from build123d import *

# Parameters (mm, degrees)
F0_R     = 1.35
F1_DEPTH = 29.5
F2_DEPTH = 37
F3_R     = 3
F4_R     = 10
F5_SIZE  = 10
F6_R     = 1.5
F7_DEPTH = 25


with BuildPart() as f1:
    # F0 (on Top) → F1 (new body)
    with BuildSketch(Plane.XY):
        with BuildLine():
            Line((-1.6, 2.8), (1.6, 2.8))
            Line((1.6, 2.8), (3.0028275917, 7.4646537393))
            ThreePointArc((3.0028275917, 7.4646537393), (0, 5.85035927), (-3.0028275917, 7.4646537393))
            Line((-3.0028275917, 7.4646537393), (-1.6, 2.8))
        make_face()
        with BuildLine():
            ThreePointArc((-3.0028275917, 7.4646537393), (0, 5.85035927), (3.0028275917, 7.4646537393))
            Line((3.0028275917, 7.4646537393), (3.6, 9.45035927))
            ThreePointArc((3.6, 9.45035927), (0, 13.05035927), (-3.6, 9.45035927))
            Line((-3.6, 9.45035927), (-3.0028275917, 7.4646537393))
        make_face()
        with Locations((0, 9.45035927)):
            Circle(F0_R, mode=Mode.SUBTRACT)
        Polygon((-15, 0), (15, 0), (15, 2.8), (1.6, 2.8), (-1.6, 2.8), (-15, 2.8), align=None)
        with BuildLine():
            ThreePointArc((-3.6, 9.45035927), (-3.4474758397, 8.4135804435), (-3.0028275917, 7.4646537393))
            Line((-3.0028275917, 7.4646537393), (-3.6, 9.45035927))
        make_face()
        with BuildLine():
            Line((3.6, 9.45035927), (3.0028275917, 7.4646537393))
            ThreePointArc((3.0028275917, 7.4646537393), (3.4474758397, 8.4135804435), (3.6, 9.45035927))
        make_face()
    extrude(amount=F1_DEPTH)

    # F0 (on Top) → F2 (join)
    with BuildSketch(Plane.XY):
        Polygon((-15, 0), (15, 0), (15, 2.8), (1.6, 2.8), (-1.6, 2.8), (-15, 2.8), align=None)
    extrude(amount=F2_DEPTH)

    # F3
    f3_edges = [f1.edges().sort_by_distance(p)[0] for p in [
        (-1.6, 2.8, 14.75),
        (1.6, 2.8, 14.75),
        (0, 2.8, 29.5),
    ]]
    fillet(f3_edges, radius=F3_R)

    # F4
    f4_edges = [f1.edges().sort_by_distance(p)[0] for p in [
        (-15, 1.4, 37),
        (15, 1.4, 37),
    ]]
    fillet(f4_edges, radius=F4_R)

    # F5
    f5_edges = [f1.edges().sort_by_distance(p)[0] for p in [
        (15, 1.4, 0),
        (-15, 1.4, 0),
    ]]
    chamfer(f5_edges, length=F5_SIZE)

    # F6 (on face) → F7 (cut)
    with BuildSketch(Plane(origin=(0, 2.8, 0), x_dir=(-1, 0, 0), z_dir=(0, 1, 0))):
        with Locations((-9, 31)):
            Circle(F6_R)
        with Locations((9, 31)):
            Circle(F6_R)
        with Locations((-9, 11)):
            Circle(F6_R)
        with Locations((9, 11)):
            Circle(F6_R)
    extrude(amount=-F7_DEPTH, mode=Mode.SUBTRACT)


solid = f1.part
Verification items for the finished model (mm, model axes). A direction names the side the tool comes from. Coordinates: 2 decimals unless noted, no trailing zeros. Write each loop counter-clockwise with the first axis right and the second up, starting at its lowest first coordinate (ties: lowest second). Pieces come first, ordered by that corner, then holes. Notation, with made-up numbers: M 33.25,88.5 L 86.25,88.5 A20 ccw 86.25,96.5 Z; hole C 27,79 d8. An arc over 180 degrees is marked long. Use a Markdown table: item, result.
Q1. Thickness scan on line 1 (Y direction, x = 0, z = 15); line 2 (Z direction, x = -9, y = 1.15); line 3 (Y direction, x = 9, z = 22). Record the ranges inside material, lowest first.
Reply:
| item | result |
|---|---|
| line 1 | y = 0 to 8.1, 10.8 to 13.05 |
| line 2 | z = 4 to 9.5, 12.5 to 29.5, 32.5 to 36.17 |
| line 3 | y = 0 to 2.8 |
Q2. Sectioned sample at B-B, the plane x = 0. Record the boundary of the cut face in (y, z), plus the area to 3 significant figures.
Reply:
| item | result |
|---|---|
| outline | M 0,0 L 8.1,0 L 8.1,29.5 L 5.8,29.5 A3 cw 2.8,32.5 L 2.8,37 L 0,37 Z; M 10.8,0 L 13.05,0 L 13.05,29.5 L 10.8,29.5 Z |
| area | 328 mm² |
Q3. Sectioned sample at D-D, the plane x = -8. Record the boundary of the cut face in (y, z).
Reply:
| item | result |
|---|---|
| outline | M 0,3 L 2.8,3 L 2.8,9.88 L 0,9.88 Z; M 0,12.12 L 2.8,12.12 L 2.8,29.88 L 0,29.88 Z; M 0,32.12 L 2.8,32.12 L 2.8,36.54 L 0,36.54 Z |
Q4. Sectioned sample at C-C, the plane z = 5. Record the boundary of the cut face in (x, y).
Reply:
| item | result |
|---|---|
| outline | M -10,0 L 10,0 L 10,2.8 L 5.63,2.8 A3 cw 2.76,6.66 L 3,7.46 A3.6 ccw long -3,7.46 L -2.76,6.66 A3 cw -5.63,2.8 L -10,2.8 Z; hole C 0,9.45 d2.7 |
Q5. Draft check along Z on faces 3 (the face through (-7.89, 1.42, 32.01)), 4 (the face through (-10, 1, 5)), 5 (the face through (2.88, 7.06, 14.54)). Enter one of: +Z half, -Z half, draft (parallel to the pull), parting line (faces both ways), or undercut.
Reply:
| item | result |
|---|---|
| face 3 | undercut |
| face 4 | -Z half |
| face 5 | draft |
Q6. Go/stop test with flat-tipped pins: P1, Ø2.5, axis at x = -9, z = 11, coming from the -Y side; P2, Ø2, axis at x = -0.5, y = 8.5, coming from the +Z side; P3, Ø4, axis at x = -9, z = 31, coming from the +Y side; P4, Ø1.5, axis at y = 4, z = 17, coming from the +X side. Record where each tip stops, or that it passes through.
Reply:
| item | result |
|---|---|
| P1 | passes through |
| P2 | stops at z = 29.5 |
| P3 | stops at y = 2.8 |
| P4 | stops at x = 4.05 |
Q7. Set-up check for faces 1 (the face through (12.15, 1.42, 33.99)), 2 (the face through (-0.1, 7.9, 29.5)): record each of +Z, -Z, +X, -X, +Y, -Y from which the full face is reachable in a straight line by a thin tool's end or side.
Reply:
| item | result |
|---|---|
| face 1 | +Z, +X, +Y, -Y |
| face 2 | +Z, +X, -X, +Y |
Q8. Sectioned sample at A-A, the plane z = 11. Record the boundary of the cut face in (x, y).
Reply:
| item | result |
|---|---|
| outline | M -15,0 L -10.5,0 L -10.5,2.8 L -15,2.8 Z; M -7.5,0 L 7.5,0 L 7.5,2.8 L 5.63,2.8 A3 cw 2.76,6.66 L 3,7.46 A3.6 ccw long -3,7.46 L -2.76,6.66 A3 cw -5.63,2.8 L -7.5,2.8 Z; M 10.5,0 L 15,0 L 15,2.8 L 10.5,2.8 Z; hole C 0,9.45 d2.7 |
